Autodesk Inventor part; units mm, degrees
ref_plane "YZ Plane" through (0, 0, 0) normal (1, 0, 0) x (0, 1, 0)
ref_plane "XZ Plane" through (0, 0, 0) normal (0, 1, 0) x (-1, 0, 0)
ref_plane "XY Plane" through (0, 0, 0) normal (0, 0, 1) x (1, 0, 0)
sketch "Boceto1" plane through (0, 0, 0) normal (0, 0, 1) x (1, 0, 0)
  line L0 (0, 0) -> (0, 50)
  line L1 (0, 50) -> (6.2, 50)
  line L2 (6.2, 50) -> (6.2, 28.5)
  line L3 (6.2, 28.5) -> (15.8, 28.5)
  line L4 (15.8, 28.5) -> (15.8, 21)
  line L5 (18.8, 18) -> (22.3, 18)
  line L6 (22.3, 18) -> (22.3, 21.9094) construction
  line L7 (41.2, 0) -> (0, 0)
  arc A0 (15.8, 21) -> (18.8, 18) centre (18.8, 21) ccw
  line L8 (22.3, 18) -> (28.4018, 18) construction
  line L9 (28.7, 21) -> (24.0321, 21)
  line L10 (22.3, 18) -> (24.0321, 21)
  line L11 (22.3, 18) -> (25.7641, 18) construction
  line L12 (59.327, 18) -> (29.2282, 18) construction
  line L13 (31.7, 18) -> (31.7, 21) construction
  line L14 (31.7, 18) -> (28.7, 21)
  line L15 (31.7, 18) -> (35.9426, 18) construction
  line L16 (31.7, 18) -> (41.2, 18) construction
  line L17 (41.2, 15.8) -> (41.2, 0)
  line L18 (31.7, 18) -> (31.7, 0)
  line L19 (31.7, 15.8) -> (41.2, 15.8)
  line L20 (22.3, 18) -> (22.3, 0)
  point P0 (15.8, 18)
  dimension "d0" = 50
  dimension "d1" = 6.2
  dimension "d2" = 9.6
  dimension "d3" = 28.5
  dimension "d4" = 6.5
  dimension "d5" = 3
  dimension "d8" = 18
  dimension "d10" = 21
  dimension "d11" = 60
  dimension "d12" = 18
  dimension "d14" = 9.4
  dimension "d15" = 135
  dimension "d16" = 9.5
  dimension "d17" = 41.2
  dimension "d18" = 15.8
revolve "Revolución1" add sketch "Boceto1" angle 360 about axis through (41.2, 0, 0) along (-1, 0, 0)
sketch "Boceto2" plane through (0, 0, 0) normal (-1, 0, 0) x (0, 0, 1)
  circle A0 centre (0, 0) radius 28.5
  point P0 (0, 0)
hole "Agujero1" at (0, 0, 0) direction (1, 0, 0) diameter 20 end through all counterbore diameter 44.5 counterbore depth 9.5
sketch "Boceto3" plane through (0, 0, 0) normal (-1, 0, 0) x (0, 0, 1)
  point P0 (0, 0)
  point P1 (0, 43)
  point P2 (-37.2391, 21.5)
  point P3 (-37.2391, -21.5)
  point P4 (0, -43)
  point P5 (37.2391, -21.5)
  point P6 (37.2391, 21.5)
  dimension "d27" = 43
  dimension "d37" = 360
hole "Agujero2" at (0, 43, 0) at (0, 21.5, 37.2391) at (0, -21.5, 37.2391) at (0, -43, 0) at (0, -21.5, -37.2391) at (0, 21.5, -37.2391) direction (1, 0, 0) diameter 7.9 end through all
thread "Rosca1"
fillet "Empalme1" radius 3 1 edges at (9.5, 0, -22.25)
properties part number "Lab15_A01209499" material "Acero, carbono"
Could you check a few things on this model? Use its own coordinates, in mm. A direction names the side the tool comes from. Round coordinates to 2 decimals unless told otherwise and drop trailing zeros. Order: outer loops, then holes, each group sorted by start corner. A loop starts at its lowest first (then second) coordinate and runs counter-clockwise, first axis right, second up.
Q1. Please list where these lines run through material, in increasing order: probe 1 along Y at (x, z) = (1.75, 0); probe 2 along X at (y, z) = (-19, -18); probe 3 along X at (y, z) = (11.5, 30.5).
Geometry says:
probe 1: y = -50 to -46.95, -39.05 to -22.25, 22.25 to 39.05, 46.95 to 50
probe 2: x = 0 to 15.8
probe 3: x = 0 to 6.2
Q2. Which directions (+Z, -Z, +X, -X, +Y, -Y) give clear straight access to the entire face, cutting with the end or side of a thin tool? Please do faces 1 (the face through (11.067, 26.327, -10.916)), 2 (the face through (20.574, -2.343, 17.847)), 3 (the face through (3.14, 23.01, -33.59)).
Geometry says:
face 1: +X
face 2: none
face 3: +X, -X
Q3. Imagine slicing it at B-B, the plane x = 17. List the corners of the cut face in (y, z) for me, then the cut area to 3 significant figures.
Geometry says:
outline: circle Ø37.2 at (0, 0); hole circle Ø20 at (0, 0)
area: 773 mm2
Q4. Thinking about a two-plate mould opening in Y: for faces 4 (the face through (3.296, -15.038, -16.399)), 5 (the face through (15.8, -13, 17)), 6 (the face through (3.14, -19.99, -33.59)), 7 (the face through (36.52, -12.54, -9.61)), which applies, released by +Y, released by -Y, zero draft, split by the parting line, or undercut?
Geometry says:
face 4: undercut
face 5: zero draft
face 6: undercut
face 7: split by the parting line
Q5. I'm going to push flat-ended pins straight in: P1, Ø11, axis at y = 9, z = 2, coming from the +X side; P2, Ø1.5, axis at x = 10.5, z = -10.5, coming from the +Y side; P3, Ø10, axis at y = 3, z = -2, coming from the +X side; P4, Ø1, axis at x = 24.5, z = 7.5, coming from the +Y side. Where does each tip first touch, or does it pass through?
Geometry says:
P1: stops at x = 41.2
P2: stops at y = 26.78
P3: passes through
P4: stops at y = 19.8
Q6. Imagine slicing it at D-D, the plane y = -41. List the corners of the cut face in (x, z) for me, then the cut area to 3 significant figures.
Geometry says:
outline: (0, -28.62) - (6.2, -28.62) - (6.2, -3.41) - (0, -3.41) - close; (0, 3.41) - (6.2, 3.41) - (6.2, 28.62) - (0, 28.62) - close
area: 313 mm2
Q7. Imagine slicing it at C-C, the plane z = 0. State how many separate pieces and enclosed holes the cut face has, then the cut area to 3 significant figures.
Geometry says:
separate pieces: 4
enclosed holes: 0
area: 935 mm2
